Autodesk Inventor part; units mm, degrees
ref_plane "YZ Plane" through (0, 0, 0) normal (1, 0, 0) x (0, 1, 0)
ref_plane "XZ Plane" through (0, 0, 0) normal (0, 1, 0) x (-1, 0, 0)
ref_plane "XY Plane" through (0, 0, 0) normal (0, 0, 1) x (1, 0, 0)
sketch "Sketch1" plane through (0, 0, 0) normal (0, 0, 1) x (1, 0, 0)
  line L0 (0, 0) -> (0, 4438.8737)
  line L1 (0, 4438.8737) -> (100, 4438.8737)
  line L2 (100, 4438.8737) -> (200, 0)
  line L3 (200, 0) -> (0, 0)
  circle A0 centre (0, 0) radius 30
  line L4 (0, 1479.6246) -> (166.6667, 1479.6246)
  line L5 (0, 2959.2492) -> (133.3333, 2959.2492)
  circle A1 centre (0, 1479.6246) radius 30
  circle A2 centre (0, 2959.2492) radius 30
  line L6 (190.4255, 425) -> (120.4255, 425)
  line L7 (120.4255, 425) -> (120.4255, 430)
  line L8 (120.4255, 430) -> (190.4255, 430)
  line L9 (190.4255, 430) -> (190.4255, 425)
  line L10 (109.1642, 929.8732) -> (179.1642, 929.8732)
  line L11 (179.1642, 924.8732) -> (109.1642, 924.8732)
  line L12 (109.1642, 924.8732) -> (109.1642, 929.8732)
  line L13 (179.1642, 929.8732) -> (179.1642, 924.8732)
  line L14 (97.903, 1429.7463) -> (167.903, 1429.7463)
  line L15 (167.903, 1424.7463) -> (97.903, 1424.7463)
  line L16 (97.903, 1424.7463) -> (97.903, 1429.7463)
  line L17 (167.903, 1429.7463) -> (167.903, 1424.7463)
  line L18 (86.6417, 1929.6195) -> (156.6417, 1929.6195)
  line L19 (156.6417, 1924.6195) -> (86.6417, 1924.6195)
  line L20 (86.6417, 1924.6195) -> (86.6417, 1929.6195)
  line L21 (156.6417, 1929.6195) -> (156.6417, 1924.6195)
  line L22 (75.3805, 2429.4927) -> (145.3805, 2429.4927)
  line L23 (145.3805, 2424.4927) -> (75.3805, 2424.4927)
  line L24 (75.3805, 2424.4927) -> (75.3805, 2429.4927)
  line L25 (145.3805, 2429.4927) -> (145.3805, 2424.4927)
  line L26 (64.1192, 2929.3658) -> (134.1192, 2929.3658)
  line L27 (134.1192, 2924.3658) -> (64.1192, 2924.3658)
  line L28 (64.1192, 2924.3658) -> (64.1192, 2929.3658)
  line L29 (134.1192, 2929.3658) -> (134.1192, 2924.3658)
  line L30 (52.8579, 3429.239) -> (122.8579, 3429.239)
  line L31 (122.8579, 3424.239) -> (52.8579, 3424.239)
  line L32 (52.8579, 3424.239) -> (52.8579, 3429.239)
  line L33 (122.8579, 3429.239) -> (122.8579, 3424.239)
  line L34 (41.5967, 3929.1122) -> (111.5967, 3929.1122)
  line L35 (111.5967, 3924.1122) -> (41.5967, 3924.1122)
  line L36 (41.5967, 3924.1122) -> (41.5967, 3929.1122)
  line L37 (111.5967, 3929.1122) -> (111.5967, 3924.1122)
  line L38 (0, 1629.6246) -> (163.2874, 1629.6246)
  line L39 (0, 3039.2492) -> (131.5311, 3039.2492)
  point P0 (30, 2959.2492)
  point P1 (0, 2929.2492)
  point P2 (0, 1509.6246)
  point P3 (0, 1449.6246)
  point P4 (0, 30)
  point P5 (30, 0)
  point P6 (190.3129, 430)
  point P7 (179.0516, 929.8732)
  point P8 (167.7903, 1429.7463)
  point P9 (30, 1479.6246)
  point P10 (156.5291, 1929.6195)
  point P11 (145.2678, 2429.4927)
  point P12 (134.0066, 2929.3658)
  point P13 (0, 2989.2492)
  dimension "d65" = 100
  dimension "d67" = 200
  dimension "d68" = 60
  dimension "d69" = 1480
  dimension "d70" = 1480
  dimension "d71" = 1480
  dimension "d72" = 5
  dimension "d73" = 70
  dimension "d74" = 430
  dimension "d77" = 500
  dimension "d82" = 80
  dimension "d83" = 150
extrude "Plate3" add sketch "Sketch1" along normal blind 4 contours L39 L2 L5 A2 L0 | L5 L2 L26 L28 L27 L22 L24 L23 L18 L20 L19 L38 L0 A2 | L38 L2 L4 A1 L0
chamfer "Corner Chamfer2" distance 3 angle 45 6 edges at (156.6417, 1924.6195, 2) (156.5291, 1929.6195, 2) (145.3805, 2424.4927, 2) (145.2678, 2429.4927, 2) (134.1192, 2924.3658, 2) (134.0066, 2929.3658, 2)
equation "\"BendRadius\" = Thickness"
equation "\"BendReliefWidth\" = Thickness"
equation "\"BendReliefDepth\" = 0.5 * Thickness"
equation "\"CornerReliefSize\" = 4 * Thickness"
equation "\"MinimumRemnant\" = 2 * Thickness"
equation "\"TransitionRadius\" = BendRadius"
equation "\"JacobiRadiusSize\" = BendRadius"
equation "\"GapSize\" = Thickness"
properties part number "0711 GBK Center rib 2" material "Steel"
Build history of the part. All positions in model axes, mm. Round coordinates to 2 decimals unless told otherwise and drop trailing zeros. Write each loop counter-clockwise with the first axis right and the second up, starting at its lowest first coordinate (ties: lowest second). Pieces come first, ordered by that corner, then holes. Notation, with made-up numbers: (-10.75, 9) -> (7.25, 9) arc R23 ccw to (7.25, 48) -> close; hole circle Ø1 at (38.5, -35.5). An arc over 180 degrees is marked (long way). Put each result on its own line as item: value.
Item 1: Wall check: probe 1 along Y at (x, z) = (78.5, 1.3); probe 2 along Y at (x, z) = (112.5, 0.4); probe 3 along Y at (x, z) = (74, 0.95). Give the ranges that are in metal, low to high. Write a range as from..to.
Here are the results:
probe 1: y = 1479.62..2424.49, 2429.49..2924.37, 2929.37..3039.25
probe 2: y = 1479.62..1924.62, 1929.62..2424.49, 2429.49..2924.37, 2929.37..3039.25
probe 3: y = 1479.62..2924.37, 2929.37..3039.25
Item 2: Slice it at A-A, the plane z = 2.7. Give the cut face in (x, y).
Here are the results:
outline: (0, 1509.62) arc R30 cw to (30, 1479.62) -> (166.67, 1479.62) -> (156.71, 1921.62) -> (153.64, 1924.62) -> (86.64, 1924.62) -> (86.64, 1929.62) -> (153.53, 1929.62) -> (156.46, 1932.62) -> (145.45, 2421.49) -> (142.38, 2424.49) -> (75.38, 2424.49) -> (75.38, 2429.49) -> (142.27, 2429.49) -> (145.2, 2432.49) -> (134.19, 2921.37) -> (131.12, 2924.37) -> (64.12, 2924.37) -> (64.12, 2929.37) -> (131.01, 2929.37) -> (133.94, 2932.37) -> (131.53, 3039.25) -> (0, 3039.25) -> (0, 2989.25) arc R30 cw to (0, 2929.25) -> close
Item 3: Slice it at C-C, the plane y = 1772.5. Give the cut face in (x, z).
Here are the results:
outline: (0, 0) -> (160.07, 0) -> (160.07, 4) -> (0, 4) -> close
Item 4: Two-plate mould, pull along Y, no slides. Class faces 1 (the face through (29.993, 2959.909, 1.972)), 2 (the face through (20.98, 1501.07, 1.97)), 3 (the face through (82, 2270, 4)): pulls with the +Y half, pulls with the -Y half, needs draft (parallel to the pull), parting line crosses it, or undercut.
Here are the results:
face 1: undercut
face 2: pulls with the -Y half
face 3: needs draft
Item 5: Flat gauge pins, fed straight in: P1, Ø2, axis at y = 2928, z = 3, coming from the +X side; P2, Ø1.5, axis at y = 2569, z = 1.5, coming from the +X side; P3, Ø1.2, axis at y = 2427.5, z = 3, coming from the +X side. Where does each tip first touch, or does it go through?
Here are the results:
P1: stops at x = 64.12
P2: stops at x = 142.14
P3: stops at x = 75.38
Item 6: Slice it at B-B, the plane y = 2082. Give the cut face in (x, z), plus the area to 3 significant figures.
Here are the results:
outline: (0, 0) -> (153.1, 0) -> (153.1, 4) -> (0, 4) -> close
area: 612 mm^2
